from build123d import *

# Parameters (mm, degrees)
F1_R     = 2
F2_DEPTH = 4


with BuildPart() as f2:
    # F1 (on Front) → F2 (new body)
    with BuildSketch(Plane.XZ):
        with BuildLine():
            ThreePointArc((10, 15), (5.606602, 25.606602), (-5, 30))
            Line((-5, 30), (-10, 30))
            Line((-10, 30), (-10, 15))
            ThreePointArc((-10, 15), (-11.464466, 11.464466), (-15, 10))
            ThreePointArc((-15, 10), (-25.606602, 5.606602), (-30, -5))
            Line((-30, -5), (-30, -10))
            Line((-30, -10), (-15, -10))
            ThreePointArc((-15, -10), (-11.464466, -11.464466), (-10, -15))
            ThreePointArc((-10, -15), (-5.606602, -25.606602), (5, -30))
            Line((5, -30), (10, -30))
            Line((10, -30), (10, -15))
            ThreePointArc((10, -15), (11.464466, -11.464466), (15, -10))
            ThreePointArc((15, -10), (25.606602, -5.606602), (30, 5))
            Line((30, 5), (30, 10))
            Line((30, 10), (15, 10))
            ThreePointArc((15, 10), (11.464466, 11.464466), (10, 15))
        make_face()
        Circle(F1_R, mode=Mode.SUBTRACT)
    extrude(amount=F2_DEPTH)


solid = f2.part
Design review of the part built by this model. Coordinates are the model's own, in mm. A direction names the side the tool comes from. Coordinates: 2 decimals unless noted, no trailing zeros. Loops run counter-clockwise (first coordinate to the right, second up) from the corner with the lowest first, then second, coordinate; pieces in that order, holes last. Notation, with made-up numbers: (-31.5, -27.5) -> (25.5, -27.5) arc R27 ccw to (25.5, -7.5) -> close; hole circle Ø8 at (71, 35.25). An arc over 180 degrees is marked (long way). Use a Markdown table: item, result. Add a question column.
Item 1: We need section D-D, the plane z = -12. Write out the cut boundary in (x, y).
Item 2: The part is to be moulded in two halves that separate along Z. For faces 4 (the cylindrical face through (25.49, -1.97, -5.72)), 5 (the cylindrical face through (0, -2, -2)), 6 (the flat face through (10, -2, -23)), say which applies: +Z half, -Z half, draft (parallel to the pull), parting line (faces both ways), or undercut.
Item 3: We need section C-C, the plane x = 0. Write out the cut boundary in (y, z), and give its area (3 significant figures).
Item 4: Machinability: for faces 1 (the flat face through (-23, -2, -10)), 2 (the flat face through (7, -2, -30)), 3 (the flat face through (-10, -2, 23)), which of the approach directions +Z, -Z, +X, -X, +Y, -Y give a long, thin tool a straight path to every point of the face, cutting with its end or side? Answer none if there is none.
Item 5: Wall thickness on L1, parallel to X at y = -2.6, z = 15.5; L2, parallel to Z at x = 0, y = -1.4; L3, parallel to X at y = -2.65, z = -27: over which ranges is each line inside the solid? List them lowest first. Write a range as from..to.
Item 6: We need section B-B, the plane z = 0. Write out the cut boundary in (x, y), and give its area (3 significant figures).
Item 7: We need section A-A, the plane y = -2.35. Write out the cut boundary in (x, z), and give its area (3 significant figures).
Item 8: Clearance check with flat-ended pins moving along their axes: P1, Ø1, axis at y = -2, z = 22, coming from the +X side; P2, Ø1.5, axis at x = 0.5, z = 24, coming from the +Y side; P3, Ø1.5, axis at x = 12, y = -3, coming from the +Z side; P4, Ø1, axis at y = -2, z = 20, coming from the -X side. State where each tip first meets the part, or that it passes through.
Numbers:
| question | item | result |
|---|---|---|
| 1 | outline | (-11, -4) -> (11, -4) -> (11, 0) -> (-11, 0) -> close |
| 2 | face 4 | -Z half |
| 2 | face 5 | undercut |
| 2 | face 6 | draft |
| 3 | outline | (-4, -29.14) -> (0, -29.14) -> (0, -2) -> (-4, -2) -> close; (-4, 2) -> (0, 2) -> (0, 29.14) -> (-4, 29.14) -> close |
| 3 | area | 217 mm^2 |
| 4 | face 1 | -Z, -X, +Y, -Y |
| 4 | face 2 | -Z, +X, -X, +Y, -Y |
| 4 | face 3 | +Z, -X, +Y, -Y |
| 5 | L1 | x = -10..9.99 |
| 5 | L2 | z = -29.14..-2, 2..29.14 |
| 5 | L3 | x = -4..10 |
| 6 | outline | (-29.14, -4) -> (-2, -4) -> (-2, 0) -> (-29.14, 0) -> close; (2, -4) -> (29.14, -4) -> (29.14, 0) -> (2, 0) -> close |
| 6 | area | 217 mm^2 |
| 7 | outline | (-30, -10) -> (-15, -10) arc R5 cw to (-10, -15) arc R15 ccw to (5, -30) -> (10, -30) -> (10, -15) arc R5 cw to (15, -10) arc R15 ccw to (30, 5) -> (30, 10) -> (15, 10) arc R5 cw to (10, 15) arc R15 ccw to (-5, 30) -> (-10, 30) -> (-10, 15) arc R5 cw to (-15, 10) arc R15 ccw to (-30, -5) -> close; hole circle Ø4 at (0, 0) |
| 7 | area | 1,820 mm^2 |
| 8 | P1 | stops at x = 8.52 |
| 8 | P2 | stops at y = 0 |
| 8 | P3 | stops at z = 11.69 |
| 8 | P4 | stops at x = -10 |
